Geometry: see drawing. Coordinates: mm, zero at the bounding-box minimum. A direction names the side the tool comes from. Give positions to 0.01 mm unless a question says otherwise; leave off trailing zeros. Loops run counter-clockwise (first coordinate to the right, second up) from the corner with the lowest first, then second, coordinate; pieces in that order, holes last. Notation, with made-up numbers: (61, 50.25) - (81, 50.25) arc R6 ccw to (81, 56.25) - close; hole circle Ø2 at (76.5, 74). An arc over 180 degrees is marked (long way). Use CSV: the item, a comma, the result in double quotes. Start each with the question number.
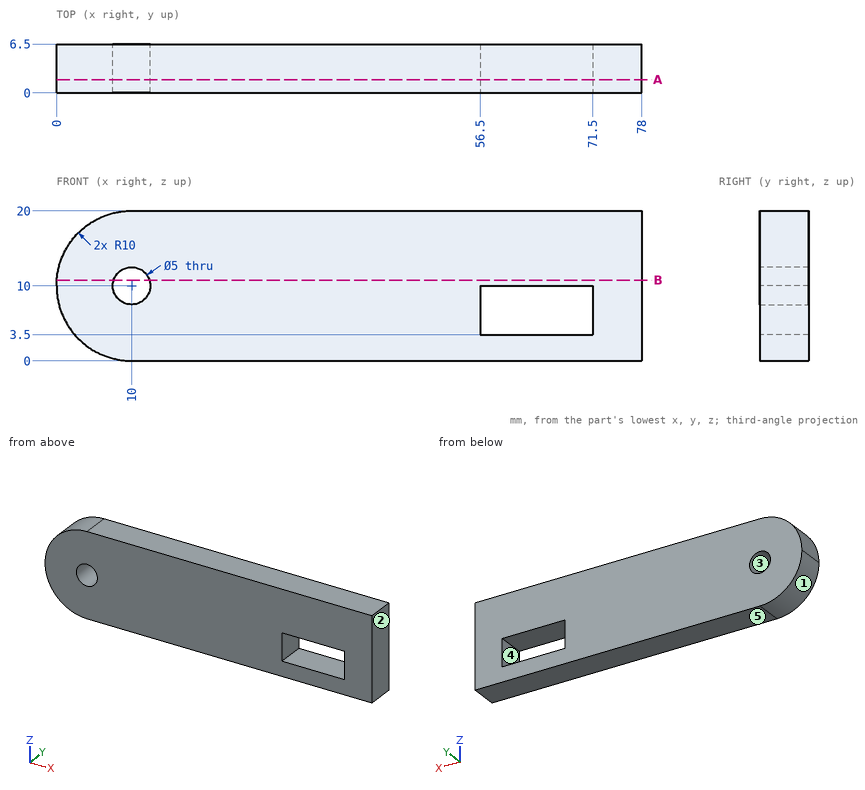
Item 1: Mould query, pull axis X, two halves, no side actions, for the marked faces 1, 2 and 3. Classes: pulls with the +X half, pulls with the -X half, needs draft (parallel to the pull), parting line crosses it, or undercut.
Item 2: Ray query, probe 1 along X at (y, z) = (3.75, 9.75); probe 2 along X at (y, z) = (2, 8); probe 3 along Z at (x, y) = (11, 1). Return the intervals inside material, ascending.
Item 3: Reachability of the marked faces 4 and 5 from +Z, -Z, +X, -X, +Y, -Y: full face, straight path, thin tool, end or side. Return the list, or none.
Item 4: Pin query (flat end, axial travel): pin 1 Ø2 at (y, z) = (4, 5.5) entering from -X. Return the tip coordinate at first contact, or that it passes through.
Item 5: Section A-A (y = 1.75). Give the number of separate pieces and of enclosed holes in the cut face, plus the area to 3 significant figures.
Item 6: Section B-B (z = 10.75). Output: boundary loops of the cut face in (x, y) (3 decimals), plus the area to 3 significant figures.
Outcome:
1,face 1,"pulls with the -X half"
1,face 2,"pulls with the +X half"
1,face 3,"undercut"
2,probe 1,"x = 0 to 7.51, 12.49 to 56.5, 71.5 to 78"
2,probe 2,"x = 0.2 to 8.5, 11.5 to 56.5, 71.5 to 78"
2,probe 3,"z = 0 to 7.71, 12.29 to 20"
3,face 4,"+Y, -Y"
3,face 5,"-Z, +X, -X, +Y, -Y"
4,pin 1,"stops at x = 0.63"
5,separate pieces,"1"
5,enclosed holes,"2"
5,area,"1,400 mm2"
6,outline,"(0.028, 0) - (7.615, 0) - (7.615, 6.5) - (0.028, 6.5) - close; (12.385, 0) - (78, 0) - (78, 6.5) - (12.385, 6.5) - close"
6,area,"476 mm2"
